Part print with two shaded views. Sizes in mm from the minimum x, y, z corner. A direction names the side the tool comes from. Round coordinates to 2 decimals unless told otherwise and drop trailing zeros. Write each loop counter-clockwise with the first axis right and the second up, starting at its lowest first coordinate (ties: lowest second). Pieces come first, ordered by that corner, then holes. Notation, with made-up numbers: (-25.75, -8.75) - (29.25, -8.75) arc R14 cw to (29.25, -1.75) - close; hole circle Ø8 at (-6, 87.5). An arc over 180 degrees is marked (long way). Use one line per item in the form item = value. Start each with the question number.
Item 1: Pin check, flat tips, straight feed: pin 1 (8 mm diameter, centred on x = 55, y = 7, fed in from +Z); pin 2 (1 mm diameter, centred on x = 56.5, z = 60.5, fed in from +Y); pin 3 (8 mm diameter, centred on x = 17, z = 14, fed in from +Y). Stop position of each tip, or through.
Item 2: Tool access for the marked faces 4, 5, 6, 7 and 8: list every direction of +Z, -Z, +X, -X, +Y, -Y with a clear straight run to the whole face (end or side of a thin tool).
Item 3: Band-saw the part on A-A, the plane z = 31. Give the number of separate pieces and of enclosed holes in the cut face, and give its area (3 significant figures).
Item 4: Pull direction Y, two halves, no side cores. Call the marked faces 1, 2 and 3: +Y half, -Y half, draft (parallel to the pull), parting line (faces both ways), or undercut.
Item 5: Band-saw the part on C-C, the plane y = 47.75. List the corners of the cut face in (x, z) (1 decimal), and give its area (3 significant figures).
Item 6: Band-saw the part on D-D, the plane x = 42.5. List the corners of the cut face in (y, z), and give its area (3 significant figures).
Item 7: Drill centre lines: L1, parallel to X at y = 47, z = 17; L2, parallel to Y at x = 56.5, z = 94.5 (1 decimal); L3, parallel to Y at x = 61, z = 29. Where is each one in solid material? Low to high.
Item 8: Band-saw the part on B-B, the plane x = 88. List the corners of the cut face in (y, z).
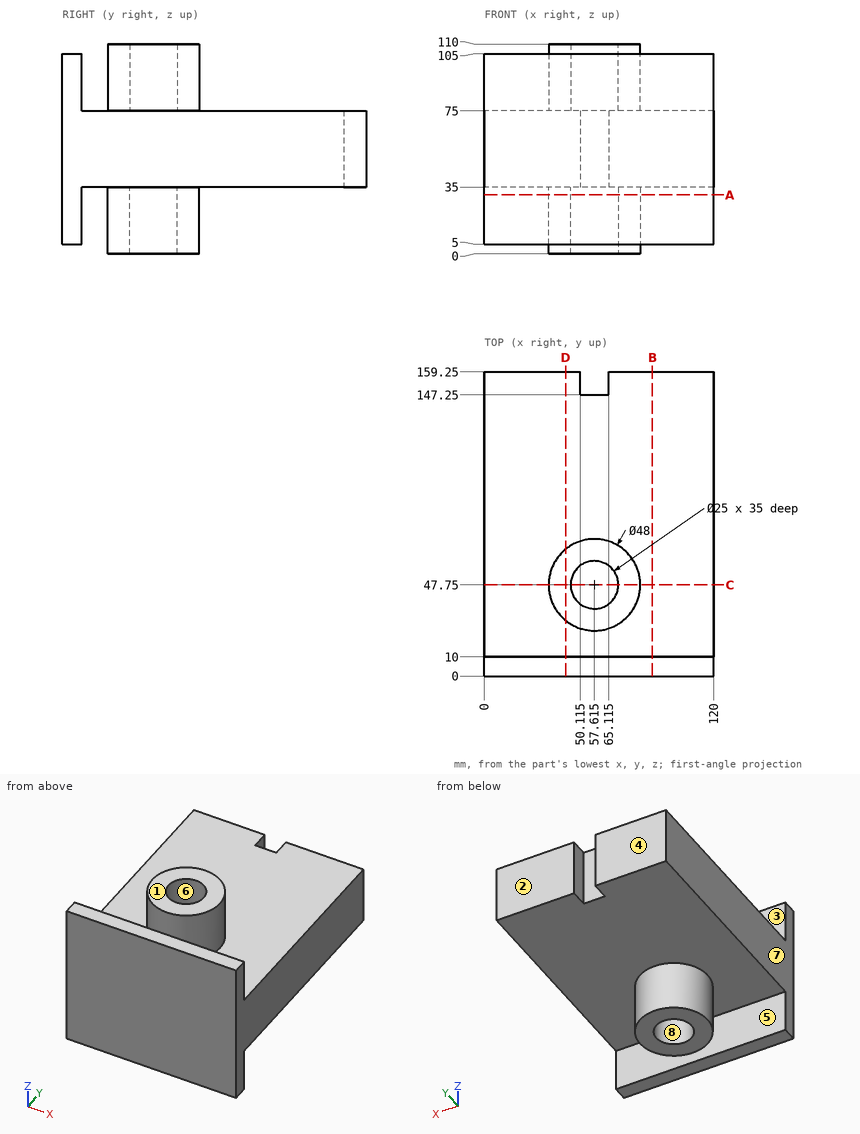
Determined:
q1.pin_1 = 105
q1.pin_2 = 147.25
q1.pin_3 = 10
q2.face_4 = +Z, -Z, +X, -X, +Y
q2.face_5 = -Z, +X, -X
q2.face_6 = +Z
q2.face_7 = +Z, -Z, -X, +Y, -Y
q2.face_8 = -Z
q3.separate_pieces = 2
q3.enclosed_holes = 1
q3.area = 2,520 mm²
q4.face_1 = draft
q4.face_2 = +Y half
q4.face_3 = undercut
q5.outline = (0, 35) - (33.6, 35) - (33.6, 0) - (45.1, 0) - (45.1, 35) - (70.1, 35) - (70.1, 0) - (81.6, 0) - (81.6, 35) - (120, 35) - (120, 75) - (81.6, 75) - (81.6, 110) - (70.1, 110) - (70.1, 75) - (45.1, 75) - (45.1, 110) - (33.6, 110) - (33.6, 75) - (0, 75) - close
q5.area = 6,410 mm²
q6.outline = (0, 5) - (10, 5) - (10, 35) - (29.11, 35) - (29.11, 0) - (66.39, 0) - (66.39, 35) - (159.25, 35) - (159.25, 75) - (66.39, 75) - (66.39, 110) - (29.11, 110) - (29.11, 75) - (10, 75) - (10, 105) - (0, 105) - close
q6.area = 9,580 mm²
q7.L1 = 33.63 to 45.14, 70.09 to 81.6
q7.L2 = 0 to 10, 23.8 to 35.3, 60.2 to 71.7
q7.L3 = 0 to 10, 23.99 to 35.72, 59.78 to 71.51
q8.outline = (0, 5) - (10, 5) - (10, 35) - (159.25, 35) - (159.25, 75) - (10, 75) - (10, 105) - (0, 105) - close
